from build123d import *

# Parameters (mm, degrees)
SKETCH2_R          = 2.5
CUT_EXTRUDE1_DEPTH = 33.5
CIRPATTERN1_COUNT  = 8


with BuildPart() as part:
    # Sketch1 → Revolve1 (revolve)
    with BuildSketch(Plane.XY):
        Polygon((-3.5, 29), (3.5, 29), (3.5, 32.5), (5, 32.5), (5, 22.5), (3.5, 22.5), (3.5, 26), (-3.5, 26), (-3.5, 22.5), (-5, 22.5), (-5, 32.5), (-3.5, 32.5), align=None)
    revolve(axis=Axis((-5.608551002, 0, 0), (1, 0, 0)))

    # Sketch2 → Cut-Extrude1 (cut, through all)
    with BuildSketch(Plane(origin=(0, 0, 0), x_dir=(1, 0, 0), z_dir=(0, 1, 0))):
        Circle(SKETCH2_R)
    cut_extrude1 = extrude(amount=CUT_EXTRUDE1_DEPTH, mode=Mode.SUBTRACT)

    # CirPattern1: Cut-Extrude1 ×8 about axis
    cirpattern1_axis = Axis((-5.608551002, 0, 0), (-1, 0, 0))
    for i in range(1, CIRPATTERN1_COUNT):
        add(cut_extrude1.rotate(cirpattern1_axis, i * 360 / CIRPATTERN1_COUNT), mode=Mode.SUBTRACT)


solid = part.part
Geometry check sheet. Reference: the model listing, model coordinates, mm. A direction names the side the tool comes from. Coordinates: 2 decimals unless noted, no trailing zeros. Order: outer loops, then holes, each group sorted by start corner. A loop starts at its lowest first (then second) coordinate and runs counter-clockwise, first axis right, second up. Notation, with made-up numbers: (-34.5, 3) - (23.5, 3) arc R10 ccw to (23.5, 13) - close; hole circle Ø11 at (48.5, 48.5). An arc over 180 degrees is marked (long way). Answer in a Markdown table with one row per item. Add a question column.
1) Material ranges on line 1 along X through (y, z) = (-22.5, 6.5); line 2 along Z through (x, y) = (-3.8, 0); line 3 along X through (y, z) = (0, 27.9), recorded low to high. Write a range as [from, to].
2) Cross-section at D-D, the plane y = 12.5. Record the cut outline in (x, z).
3) Set-up check for faces 1 (the flat face through (3.5, 11.7, 19.4)), 2 (the cylindrical face through (2.385, -0.751, -27.419)): record each of +Z, -Z, +X, -X, +Y, -Y from which the full face is reachable in a straight line by a thin tool's end or side.
4) Gauge pin test, flat ends, axial feed: P1, Ø5, axis at x = -3, z = 10, coming from the -Y side; P2, Ø4, axis at x = 3, z = 22, coming from the -Y side; P3, Ø1, axis at x = -4, y = -0.5, coming from the +Z side. Record the tip position at first contact, or that the pin passes through.
5) Release check for a two-part mould opening along X. For faces 3 (the flat face through (-5, -7, 22)), 4 (the flat face through (5, 7, 22)), 5 (the cylindrical face through (-1.984, 18.313, 20.464)), 6 (the cylindrical face through (4.26, 31, 9.76)) record: +X half, -X half, draft (parallel to the pull), parting line (faces both ways), or undercut.
6) Cross-section at A-A, the plane z = 0. State how many separate pieces and enclosed holes the cut face has, then the cut area to 3 significant figures.
Check result:
| question | item | result |
|---|---|---|
| 1 | line 1 | x = [-5, -3.5], [3.5, 5] |
| 1 | line 2 | z = [-32.5, -22.5], [22.5, 32.5] |
| 1 | line 3 | x = [-5, -2.5], [2.5, 5] |
| 2 | outline | (-5, -30) - (-3.5, -30) - (-3.5, -26.17) - (3.5, -26.17) - (3.5, -30) - (5, -30) - (5, -18.71) - (3.5, -18.71) - (3.5, -22.8) - (-3.5, -22.8) - (-3.5, -18.71) - (-5, -18.71) - close; (-5, 18.71) - (-3.5, 18.71) - (-3.5, 22.8) - (3.5, 22.8) - (3.5, 18.71) - (5, 18.71) - (5, 30) - (3.5, 30) - (3.5, 26.17) - (-3.5, 26.17) - (-3.5, 30) - (-5, 30) - close |
| 3 | face 1 | none |
| 3 | face 2 | +Z, -Z |
| 4 | P1 | stops at y = -31.61 |
| 4 | P2 | stops at y = -25.57 |
| 4 | P3 | stops at z = 32.5 |
| 5 | face 3 | -X half |
| 5 | face 4 | +X half |
| 5 | face 5 | undercut |
| 5 | face 6 | draft |
| 6 | separate pieces | 4 |
| 6 | enclosed holes | 0 |
| 6 | area | 72.0 mm² |
